Can you work these out from the model? Positions are in its coordinate system, mm. A direction names the side the tool comes from. Coordinates: 2 decimals unless noted, no trailing zeros. Write each loop counter-clockwise with the first axis right and the second up, starting at its lowest first coordinate (ties: lowest second). Pieces come first, ordered by that corner, then holes. Notation, with made-up numbers: (21, 6.25) - (41, 6.25) arc R11 cw to (41, 17.25) - close; hole circle Ø10 at (-23, 30.25). An arc over 180 degrees is marked (long way). Use one line per item in the form item = value. Start each with the question number.
(1) If we section it at B-B on y = -14.75: Give the number of separate pieces and of enclosed holes in the cut face, then the cut area to 3 significant figures.
(2) If I drill on probe 1 along Z at (x, y) = (-10, -13.75); probe 2 along Z at (x, y) = (4, -11.25); probe 3 along X at (y, z) = (-1, 25.5), over which ranges is the centre line in solid material (lowest first)? Write a range as from..to.
(3) For pin 1 Ø10 at (y, z) = (-5.5, 29.5) entering from +X; pin 2 Ø3 at (x, z) = (-10, 6) entering from -Y; pin 3 Ø5 at (y, z) = (-12.5, -3.5) entering from -X; pin 4 Ø8 at (x, z) = (26.5, -1) entering from -Y, each with a flat end and sliding along its axis, tell me the tip position at first contact or that it passes through.
(4) On a 3-axis mill with a long thin cutter (end or side, diameter ignored), from which of +Z, -Z, +X, -X, +Y, -Y can I reach the whole of each face in a straight line? I mean faces 1 (the face through (31.664, -9, 21)), 2 (the face through (0, -12, -4)), 3 (the face through (-8.636, -9, 21)), 4 (the face through (31.664, -9, 3)). Say none if no direction works.
(5) Thinking about a two-plate mould opening in X: for faces 5 (the face through (-14.785, -15.558, 6.332)), 6 (the face through (-8.636, -9, 3)), 7 (the face through (2, -9, -4)), 8 (the face through (-12, 0.213, 6)), which applies, pulls with the +X half, pulls with the -X half, needs draft (parallel to the pull), parting line crosses it, or undercut?
(6) If we section it at A-A on z = 8.5: Please give me the cut outline in (x, y).
```python
from build123d import *

# Parameters (mm, degrees)
EXTRUDE_1_DEPTH     = 35
EXTRUDE_2_DEPTH     = 2
SKETCH_10_R         = 7
EXTRUDE_6_DEPTH     = 2
SKETCH_15_R         = 2.9
EXTRUDE_7_DEPTH     = 4
SKETCH_16_R         = 1.5
CUT_EXTRUDE_1_DEPTH = 4
SKETCH_17_W         = 2.5
SKETCH_17_H         = 18.5
EXTRUDE_9_DEPTH     = 6.85
SKETCH_19_R         = 2.5
CUT_EXTRUDE_2_DEPTH = 30.9
FILLET_1_R          = 1
FILLET_2_R          = 1
FILLET_3_R          = 1
FILLET_4_R          = 1
FILLET_5_R          = 0.5
FILLET_6_R          = 0.5
FILLET_7_R          = 0.5


with BuildPart() as part:
    # 草图1 → 凸台-拉伸1 (new body)
    with BuildSketch(Plane.XY):
        with BuildLine():
            Line((-8.135874765, 0.713393676), (31.164125235, 0.713393676))
            ThreePointArc((31.164125235, 0.713393676), (31.517678626, 0.566947067), (31.664125235, 0.213393676))
            Line((31.664125235, 0.213393676), (31.664125235, -18.286606324))
            ThreePointArc((31.664125235, -18.286606324), (31.517678626, -18.640159714), (31.164125235, -18.786606324))
            Line((31.164125235, -18.786606324), (-8.135874765, -18.786606324))
            ThreePointArc((-8.135874765, -18.786606324), (-8.489428155, -18.640159714), (-8.635874765, -18.286606324))
            Line((-8.635874765, -18.286606324), (-8.635874765, 0.213393676))
            ThreePointArc((-8.635874765, 0.213393676), (-8.489428155, 0.566947067), (-8.135874765, 0.713393676))
        make_face()
    extrude(amount=EXTRUDE_1_DEPTH)

    # 草图2 → 凸台-拉伸2 (add)
    with BuildSketch(Plane(origin=(0, 0, 0), x_dir=(-1, 0, 0), z_dir=(0, 0, -1))):
        with BuildLine():
            Line((-25.664125235, -18.286606324), (-25.664125235, 0.213393676))
            ThreePointArc((-25.664125235, 0.213393676), (-25.517678626, 0.566947067), (-25.164125235, 0.713393676))
            Line((-25.164125235, 0.713393676), (-1.114125235, 0.713393676))
            ThreePointArc((-1.114125235, 0.713393676), (8.635874765, -9.036606324), (-1.114125235, -18.786606324))
            Line((-1.114125235, -18.786606324), (-25.164125235, -18.786606324))
            ThreePointArc((-25.164125235, -18.786606324), (-25.517678626, -18.640159714), (-25.664125235, -18.286606324))
        make_face()
    extrude(amount=EXTRUDE_2_DEPTH)

    # 草图10 → 凸台-拉伸6 (add)
    with BuildSketch(Plane(origin=(0, 0, -2), x_dir=(-1, 0, 0), z_dir=(0, 0, -1))):
        with Locations((-1.664125235, -9.036606324)):
            Circle(SKETCH_10_R)
    extrude(amount=EXTRUDE_6_DEPTH)

    # 草图15 → 凸台-拉伸7 (add)
    with BuildSketch(Plane(origin=(0, 0, -4), x_dir=(-1, 0, 0), z_dir=(0, 0, -1))):
        with Locations((-1.664125235, -9.036606324)):
            Circle(SKETCH_15_R)
    extrude(amount=EXTRUDE_7_DEPTH)

    # 草图16 → 切除-拉伸1 (cut)
    with BuildSketch(Plane(origin=(0, 0, -8), x_dir=(-1, 0, 0), z_dir=(0, 0, -1))):
        with Locations((-1.664125235, -9.036606324)):
            Circle(SKETCH_16_R)
    extrude(amount=-CUT_EXTRUDE_1_DEPTH, mode=Mode.SUBTRACT)

    # 草图17 → 凸台-拉伸9 (add)
    with BuildSketch(Plane(origin=(31.664125235, 0, 0), x_dir=(0, 0, -1), z_dir=(1, 0, 0))):
        with Locations((-6.35, -9.036606324)):
            Rectangle(SKETCH_17_W, SKETCH_17_H)
    extrude_9 = extrude(amount=EXTRUDE_9_DEPTH)

    # 草图19 → 切除-拉伸2 (cut, through all)
    with BuildSketch(Plane(origin=(0, 0, 5.1), x_dir=(-1, 0, 0), z_dir=(0, 0, -1))):
        with Locations((-35.829125235, -4.036606324)):
            Circle(SKETCH_19_R)
        with Locations((-35.829125235, -14.036606324)):
            Circle(SKETCH_19_R)
    cut_extrude_2 = extrude(amount=-CUT_EXTRUDE_2_DEPTH, mode=Mode.SUBTRACT)

    # 镜向3: 凸台-拉伸9, 切除-拉伸2 across plane
    add(extrude_9.mirror(Plane.ZY.offset(-11.514125235)))
    add(cut_extrude_2.mirror(Plane.ZY.offset(-11.514125235)), mode=Mode.SUBTRACT)

    # 圆角1
    fillet_1_edges = [part.edges().sort_by_distance(p)[0] for p in [
        (38.514125235, 0.213393676, 6.35),
    ]]
    fillet(fillet_1_edges, radius=FILLET_1_R)

    # 圆角2
    fillet_2_edges = [part.edges().sort_by_distance(p)[0] for p in [
        (38.514125235, -18.286606324, 6.35),
    ]]
    fillet(fillet_2_edges, radius=FILLET_2_R)

    # 圆角3
    fillet_3_edges = [part.edges().sort_by_distance(p)[0] for p in [
        (-15.485874765, 0.213393676, 6.35),
    ]]
    fillet(fillet_3_edges, radius=FILLET_3_R)

    # 圆角4
    fillet_4_edges = [part.edges().sort_by_distance(p)[0] for p in [
        (-15.485874765, -18.286606324, 6.35),
    ]]
    fillet(fillet_4_edges, radius=FILLET_4_R)

    # 圆角5
    fillet_5_edges = [part.edges().sort_by_distance(p)[0] for p in [
        (4.564125235, -9.036606324, -8),
    ]]
    fillet(fillet_5_edges, radius=FILLET_5_R)

    # 圆角6
    fillet_6_edges = [part.edges().sort_by_distance(p)[0] for p in [
        (8.664125235, -9.036606324, -4),
    ]]
    fillet(fillet_6_edges, radius=FILLET_6_R)

    # 圆角7
    fillet_7_edges = [part.edges().sort_by_distance(p)[0] for p in [
        (13.139125235, 0.713393676, -2),
        (25.664125235, -9.036606324, -2),
        (13.139125235, -18.786606324, -2),
        (-8.635874765, -9.036606324, -2),
    ]]
    fillet(fillet_7_edges, radius=FILLET_7_R)


solid = part.part
```
Reported:
q1.separate_pieces = 3
q1.enclosed_holes = 0
q1.area = 1,500 mm2
q2.probe_1 = 5.1..7.6
q2.probe_2 = -4..35
q2.probe_3 = -8.64..31.66
q3.pin_1 = 31.66
q3.pin_2 = -18.63
q3.pin_3 = -8.45
q3.pin_4 = -18.79
q4.face_1 = +Z, +X, +Y, -Y
q4.face_2 = -Z
q4.face_3 = +Z, -X, +Y, -Y
q4.face_4 = -Z, +X, +Y, -Y
q5.face_5 = undercut
q5.face_6 = pulls with the -X half
q5.face_7 = undercut
q5.face_8 = needs draft
q6.outline = (-8.64, -18.29) arc R0.5 ccw to (-8.14, -18.79) - (31.16, -18.79) arc R0.5 ccw to (31.66, -18.29) - (31.66, 0.21) arc R0.5 ccw to (31.16, 0.71) - (-8.14, 0.71) arc R0.5 ccw to (-8.64, 0.21) - close
